Check sheet for the drawn part. Datum: minimum x, y, z corner. Units: mm. Give positions to 0.01 mm unless a question says otherwise; leave off trailing zeros. Write each loop counter-clockwise with the first axis right and the second up, starting at its lowest first coordinate (ties: lowest second). Pieces come first, ordered by that corner, then holes. Notation, with made-up numbers: M -2,-17 L 21,-17 A19 ccw 21,15 Z; hole C 29.5,36 d10. An arc over 180 degrees is marked long. Write item = value, one per line.
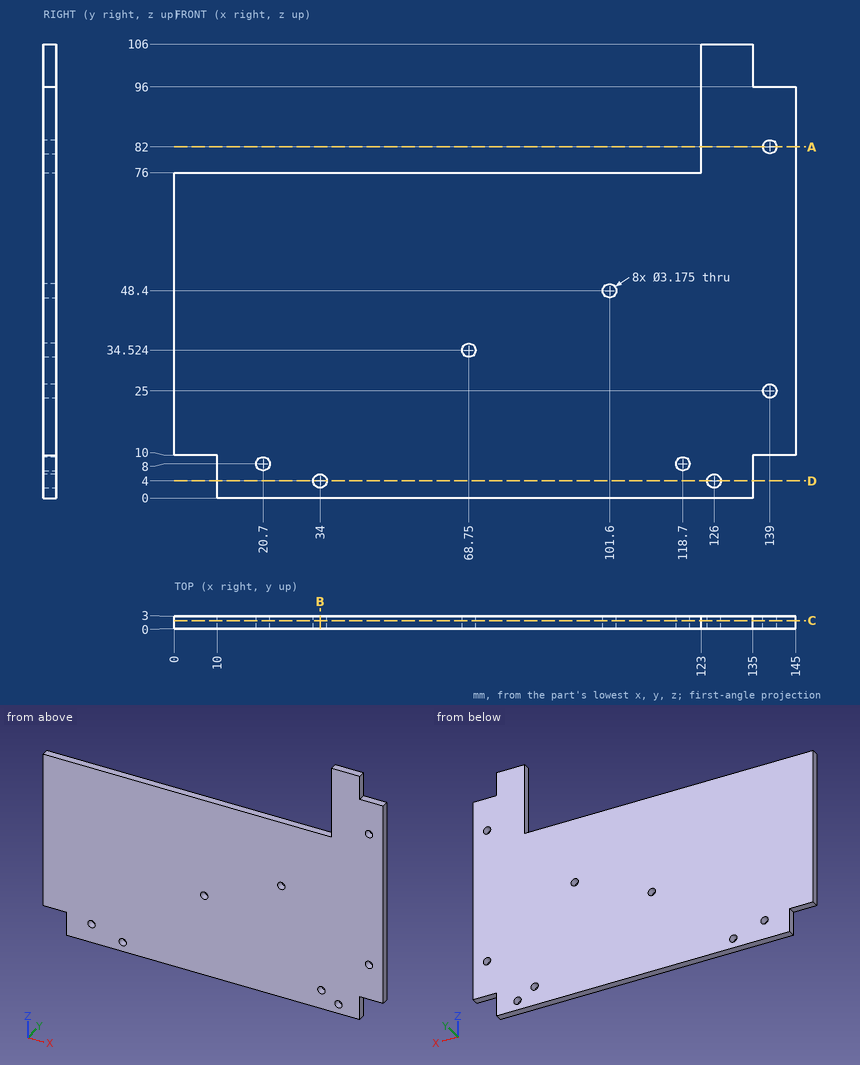
1) Material ranges on probe 1 along X at (y, z) = (0.75, 8); probe 2 along Z at (x, y) = (126, 1.8); probe 3 along Z at (x, y) = (34, 1.5), recorded low to high. Write a range as from..to.
From the geometry:
probe_1 = 10..19.11, 22.29..117.11, 120.29..135
probe_2 = 0..2.41, 5.59..106
probe_3 = 0..2.41, 5.59..76
2) Cross-section at B-B on x = 34. Record the boundary of the cut face in (y, z), plus the area to 3 significant figures.
From the geometry:
outline = M 0,0 L 3,0 L 3,2.41 L 0,2.41 Z; M 0,5.59 L 3,5.59 L 3,76 L 0,76 Z
area = 218 mm^2
3) Cross-section at D-D on z = 4. Record the boundary of the cut face in (x, y), plus the area to 3 significant figures.
From the geometry:
outline = M 10,0 L 32.41,0 L 32.41,3 L 10,3 Z; M 35.59,0 L 124.41,0 L 124.41,3 L 35.59,3 Z; M 127.59,0 L 135,0 L 135,3 L 127.59,3 Z
area = 356 mm^2
4) Depth check by flat-ended pin: P1, Ø1.5, axis at y = 1.5, z = 85.5, coming from the -X side; P2, Ø1.9, axis at x = 34, z = 4, coming from the -Y side; P3, Ø0.9, axis at y = 1, z = 101, coming from the +X side; P4, Ø0.9, axis at x = 3.5, y = 2, coming from the -Z side. Enter the tip coordinate at first touch or a pass-through.
From the geometry:
P1 = 123
P2 = through
P3 = 135
P4 = 10
5) Cross-section at C-C on y = 1.95. Count the separate pieces of the cut face and the enclosed holes in it, plus the area to 3 significant figures.
From the geometry:
separate_pieces = 1
enclosed_holes = 8
area = 11,300 mm^2
6) Cross-section at A-A on z = 82. Record the boundary of the cut face in (x, y), plus the area to 3 significant figures.
From the geometry:
outline = M 123,0 L 137.41,0 L 137.41,3 L 123,3 Z; M 140.59,0 L 145,0 L 145,3 L 140.59,3 Z
area = 56.5 mm^2
